```python
from build123d import *

# Parameters (mm, degrees)
CUT_EXTRUDE1_DEPTH          = 14
SKETCH3_R                   = 0.75
CABLE_HOLE_DEPTH            = 14
SKETCH4_R                   = 1.1303
F_5_40_SET_SCREW_HOLE_DEPTH = 3
SKETCH6_R                   = 0.8
M2_X_0_4_SCREW_HOLE_DEPTH   = 16.0000001
SKETCH7_R                   = 1.1
HOLE_FOR_CAP_SCREW_DEPTH    = 5
SKETCH8_R                   = 1.875
CUT_EXTRUDE6_DEPTH          = 2.5


with BuildPart() as part:
    # Sketch1 → Revolve1 (revolve)
    with BuildSketch(Plane.XY):
        with BuildLine():
            Line((-6.755287009, -0.373111782), (6.244712991, -0.373111782))
            Line((6.244712991, -0.373111782), (6.244712991, 7.126888218))
            ThreePointArc((6.244712991, 7.126888218), (-0.255287009, 4.626888218), (-6.755287009, 7.126888218))
            Line((-6.755287009, 7.126888218), (-6.755287009, -0.373111782))
        make_face()
    revolve(axis=Axis((-6.755287009, -0.373111782, 0), (1, 0, 0)))

    # Sketch2 → Cut-Extrude1 (cut, through all)
    with BuildSketch(Plane.ZY.offset(6.755287009)):
        with BuildLine():
            Line((1.5, 3.315769979), (1.5, 2.315769979))
            Line((1.5, 2.315769979), (-1.5, 2.315769979))
            Line((-1.5, 2.315769979), (-1.5, 3.315769979))
            Line((-1.5, 3.315769979), (-1.5, 3.415769979))
            ThreePointArc((-1.5, 3.415769979), (0, -4.448111782), (1.5, 3.415769979))
            Line((1.5, 3.415769979), (1.5, 3.315769979))
        make_face()
    extrude(amount=-CUT_EXTRUDE1_DEPTH, mode=Mode.SUBTRACT)

    # Sketch3 → cable hole (cut, through all)
    with BuildSketch(Plane(origin=(6.244712991, 0, 0), x_dir=(0, 0, -1), z_dir=(1, 0, 0))):
        with Locations((0, 3.790774627)):
            Circle(SKETCH3_R)
    extrude(amount=-CABLE_HOLE_DEPTH, mode=Mode.SUBTRACT)

    # Sketch4 → 5-40 set screw hole (cut)
    with BuildSketch(Plane(origin=(0, 7.126888218, 0), x_dir=(1, 0, 0), z_dir=(0, 1, 0))):
        with Locations((3.923493578, 0)):
            Circle(SKETCH4_R)
    extrude(amount=-F_5_40_SET_SCREW_HOLE_DEPTH, mode=Mode.SUBTRACT)

    # Sketch6 → M2 X 0.4 screw hole (cut, through all)
    with BuildSketch(Plane.XY.offset(7.5)):
        with Locations((3.762702125, 0)):
            Circle(SKETCH6_R)
        with Locations((-3.920823754, 0)):
            Circle(SKETCH6_R)
    extrude(amount=-M2_X_0_4_SCREW_HOLE_DEPTH, mode=Mode.SUBTRACT)

    # Sketch7 → hole for cap screw (cut)
    with BuildSketch(Plane.XY.offset(7.5)):
        with Locations((3.762702125, 0)):
            Circle(SKETCH7_R)
        with Locations((-3.920823754, 0)):
            Circle(SKETCH7_R)
    extrude(amount=-HOLE_FOR_CAP_SCREW_DEPTH, mode=Mode.SUBTRACT)

    # Sketch8 → Cut-Extrude6 (cut)
    with BuildSketch(Plane.XY.offset(7.5)):
        with Locations((3.762702125, 0)):
            Circle(SKETCH8_R)
        with Locations((-3.920823754, 0)):
            Circle(SKETCH8_R)
    extrude(amount=-CUT_EXTRUDE6_DEPTH, mode=Mode.SUBTRACT)


solid = part.part
```
Verification items for the finished model (mm, model axes). A direction names the side the tool comes from. Round coordinates to 2 decimals unless told otherwise and drop trailing zeros. Write each loop counter-clockwise with the first axis right and the second up, starting at its lowest first coordinate (ties: lowest second). Pieces come first, ordered by that corner, then holes. Notation, with made-up numbers: (66.25, 56) -> (123.25, 56) arc R22 ccw to (123.25, 89) -> close; hole circle Ø9 at (27.5, 31). An arc over 180 degrees is marked (long way). Write each question's results on one line, items separated by ' | '. Start each with the question number.
1. Cross-section at B-B (x = 4). Enter the section's corners in (y, z) (3 decimals), then the cut area to 3 significant figures.
2. Set-up check for faces 4 (the cylindrical face through (-5.765, -0.337, 5.685)), 5 (the flat face through (0, 2.316, 0)), 6 (the cylindrical face through (4.97, 4.95, 0.43)): record each of +Z, -Z, +X, -X, +Y, -Y from which the full face is reachable in a straight line by a thin tool's end or side.
3. Cross-section at D-D (y = 0). Count the separate pieces of the cut face and the enclosed holes in it, then the cut area to 3 significant figures.
4. Cross-section at A-A (x = -4). Enter the section's corners in (y, z) (3 decimals), then the cut area to 3 significant figures.
5. Draft check along X on faces 1 (the flat face through (6.245, -4, -3)), 2 (the flat face through (-6.755, 2.86, 0.11)), 3 (the cylindrical face through (5.5, -0.7, 5.6)). Enter one of: +X half, -X half, draft (parallel to the pull), parting line (faces both ways), or undercut.
6. Cross-section at C-C (z = 0). Enter the section's corners in (x, y), then the cut area to 3 significant figures.
7. Material ranges on probe 1 along X at (y, z) = (0, -4.9); probe 2 along X at (y, z) = (0, 4.55); probe 3 along X at (y, z) = (0, 5.45), recorded low to high. Write a range as from..to.
8. Depth check by flat-ended pin: P1, Ø1.8, axis at x = 3.92, z = 0, coming from the -Y side; P2, Ø2.5, axis at x = -3.92, y = 0, coming from the -Z side; P3, Ø0.5, axis at x = 3, y = 2.5, coming from the +Z side. Enter the tip coordinate at first touch or a pass-through.
Solutions:
1) outline: (-1.86, 5) -> (-1.86, 5.796) arc R5.983 ccw to (-0.764, -5.97) -> (-0.764, -4.056) arc R4.075 cw to (-1.074, 4.014) -> (-1.074, 5) -> close; (0.764, -5.874) arc R5.983 ccw to (5.503, -1.128) -> (4.127, -1.128) -> (4.127, -0.67) arc R0.75 cw (long way) to (4.127, 0.67) -> (4.127, 1.128) -> (5.503, 1.128) arc R5.983 ccw to (1.86, 5.551) -> (1.86, 5) -> (1.074, 5) -> (1.074, 3.809) arc R4.075 cw to (3.416, 1.5) -> (2.316, 1.5) -> (2.316, -1.5) -> (3.416, -1.5) arc R4.075 cw to (0.764, -3.913) -> close | area: 51.2 mm2
2) face 4: +Z | face 5: +X, -X | face 6: +Y
3) separate pieces: 6 | enclosed holes: 0 | area: 28.4 mm2
4) outline: (-1.873, 5) -> (-1.873, 5.553) arc R5.752 ccw to (-0.796, -5.736) -> (-0.796, -4.053) arc R4.075 cw to (-1.097, 4.01) -> (-1.097, 5) -> close; (0.796, -5.632) arc R5.752 ccw to (1.873, 5.295) -> (1.873, 5) -> (1.097, 5) -> (1.097, 3.801) arc R4.075 cw to (3.416, 1.5) -> (2.316, 1.5) -> (2.316, -1.5) -> (3.416, -1.5) arc R4.075 cw to (0.796, -3.904) -> close; hole circle Ø1.5 at (3.791, 0) | area: 46.6 mm2
5) face 1: +X half | face 2: -X half | face 3: undercut
6) outline: (-6.76, -7.87) arc R9.7 cw to (6.24, -7.87) -> (6.24, -4.45) -> (-6.76, -4.45) -> close; (-6.76, 2.32) -> (6.24, 2.32) -> (6.24, 3.04) -> (-6.76, 3.04) -> close; (-6.76, 4.54) -> (2.79, 4.54) -> (2.79, 5.12) arc R9.7 cw to (-6.76, 7.13) -> close; (5.05, 4.54) -> (6.24, 4.54) -> (6.24, 7.13) arc R9.7 cw to (5.05, 6.21) -> close | area: 40.6 mm2
7) probe 1: x = -6.76..-4.72, -3.12..2.96, 4.56..6.24 | probe 2: x = -6.76..-5.02, -2.82..2.66, 4.86..6.24 | probe 3: x = -6.76..-5.8, 5.64..6.24
8) P1: stops at y = -6.81 | P2: stops at z = -6.33 | P3: stops at z = 4.94
